Design review of the part built by this model. Coordinates are the model's own, in mm. A direction names the side the tool comes from. Give positions to 0.01 mm unless a question says otherwise; leave off trailing zeros. Write each loop counter-clockwise with the first axis right and the second up, starting at its lowest first coordinate (ties: lowest second). Pieces come first, ordered by that corner, then holes. Notation, with made-up numbers: (-16.5, -15.5) -> (42.5, -15.5) arc R17 cw to (42.5, 10.5) -> close; hole circle Ø3 at (-25.75, 3). An arc over 180 degrees is marked (long way). Return JSON: item names as keys, results as strings. Group by question number.
from build123d import *

# Parameters (mm, degrees)
SKETCH1_W               = 44.45
SKETCH1_H               = 44.45
SKETCH1_W_2             = 38.1
SKETCH1_H_2             = 38.1
BOSS_EXTRUDE1_DEPTH     = 1035.05
CUT_EXTRUDE1_DEPTH      = 1037.242373012
F_1_2_CLEARANCE_HOLE1_D = 13.49248
F_1_4_CLEARANCE_HOLE1_D = 6.7564


with BuildPart() as part:
    # Sketch1 → Boss-Extrude1 (new body)
    with BuildSketch(Plane(origin=(0, 0, 0), x_dir=(0, 0, -1), z_dir=(1, 0, 0))):
        Rectangle(SKETCH1_W, SKETCH1_H)
        Rectangle(SKETCH1_W_2, SKETCH1_H_2, mode=Mode.SUBTRACT)
    extrude(amount=BOSS_EXTRUDE1_DEPTH)

    # Sketch2 → Cut-Extrude1 (cut, through all)
    with BuildSketch(Plane.XY.offset(22.225)):
        Polygon((0, 22.225), (0, -22.225), (44.45, 22.225), align=None)
        Polygon((990.6, 22.225), (1035.05, 22.225), (1035.05, -22.225), align=None)
    extrude(amount=-CUT_EXTRUDE1_DEPTH, mode=Mode.SUBTRACT)

    # 1/2 Clearance Hole1 (through all)
    with Locations(Plane(origin=(0, -22.225, 0), x_dir=(-1, 0, 0), z_dir=(0, -1, 0))):
        with Locations((-25.4, 0), (-1009.65, 0)):
            Hole(F_1_2_CLEARANCE_HOLE1_D / 2)

    # 1/4 Clearance Hole1 (through all)
    with Locations(Plane(origin=(0, 22.225, 0), x_dir=(1, 0, 0), z_dir=(0, 1, 0))):
        with Locations((336.55, 0), (457.2, 0), (577.85, 0), (698.5, 0)):
            Hole(F_1_4_CLEARANCE_HOLE1_D / 2)


solid = part.part
Q1. Mouldability with a two-part tool opening along Y and no side actions: class faces 3 (the face through (510, 0, 19.05)), 4 (the face through (1013.136, -0.311, -19.444)), 5 (the face through (510, 0, 22.225)) as +Y half, -Y half, draft (parallel to the pull), parting line (faces both ways), or undercut.
Q2. Insertion check: pin 1 (5.5 mm diameter, centred on x = 698.5, z = 0, fed in from +Y); pin 2 (9 mm diameter, centred on x = 698.5, z = 0, fed in from -Y) (3 decimals); pin 3 (17.5 mm diameter, centred on x = 25.4, z = 0, fed in from +Y). Each pin has a flat end and moves straight along its axis. Give the tip position at first contact, or say it passes through.
Q3. Tool access review of faces 1 (the face through (511, 22.225, 0)), 2 (the face through (511, 19.05, 0)): name each direction out of +Z, -Z, +X, -X, +Y, -Y from which nothing blocks a thin tool from reaching the whole face with its end or side.
Q4. Take a section at B-B, the plane x = 798.5. Give the boundary of the cut face in (y, z) (3 decimals), plus the area to 3 significant figures.
Q5. Take a section at A-A, the plane y = 8. Give the boundary of the cut face in (x, z) (3 decimals).
Q6. For L1, parallel to Z at x = 347, y = 17.5 (3 decimals); L2, parallel to Z at x = 336, y = 21 (3 decimals), list the stretches that pass through material, from the lowest coordinate up. Write a range as from..to.
Final values:
{
 "1": {"face 3": "undercut", "face 4": "+Y half", "face 5": "draft"},
 "2": {"pin 1": "passes through", "pin 2": "stops at y = -22.225", "pin 3": "stops at y = -19.05"},
 "3": {"face 1": "+Z, -Z, +X, -X, +Y", "face 2": "+X, -X"},
 "4": {"outline": "(-22.225, -22.225) -> (22.225, -22.225) -> (22.225, 22.225) -> (-22.225, 22.225) -> close; hole (-19.05, -19.05) -> (19.05, -19.05) -> (19.05, 19.05) -> (-19.05, 19.05) -> close", "area": "524 mm²"},
 "5": {"outline": "(30.225, -22.225) -> (1004.825, -22.225) -> (1004.825, -19.05) -> (30.225, -19.05) -> close; (30.225, 19.05) -> (1004.825, 19.05) -> (1004.825, 22.225) -> (30.225, 22.225) -> close"},
 "6": {"L1": "z = -22.225..-19.05, 19.05..22.225", "L2": "z = -22.225..-3.333, 3.333..22.225"}
}
